The listing builds one solid part. Answer for the finished solid, in the listing's coordinates (mm). Face numbers are marked on the shaded views. A direction names the side the tool comes from. Round coordinates to 2 decimals unless told otherwise and drop trailing zeros. Loops run counter-clockwise (first coordinate to the right, second up) from the corner with the lowest first, then second, coordinate; pieces in that order, holes last. Notation, with made-up numbers: (12, 85.5) -> (20, 85.5) arc R29 ccw to (20, 113.5) -> close; hole circle Ø2 at (41, 45.25). An arc over 180 degrees is marked (long way). Answer in a Markdown table with one row per item. Add a question column.
```python
from build123d import *

# Parameters (mm, degrees)
BOSS_EXTRUDE1_DEPTH     = 22.4
FILLET1_R               = 2
FILLET2_R               = 5.5
BOSS_EXTRUDE2_DEPTH     = 2.73
CUT_EXTRUDE2_DEPTH      = 32.510198396
CUT_EXTRUDE2_DEPTH_BACK = 32.510198396
SKETCH3_R               = 0.95


with BuildPart() as part:
    # Sketch1 → Boss-Extrude1 (new body)
    with BuildSketch(Plane(origin=(0, 0, 0), x_dir=(1, 0, 0), z_dir=(0, 1, 0))):
        Polygon((-7.925386608, 7.925386608), (-15.2, -4.674613392), (-18.231088913, -2.924613392), (-9.94611255, 11.425386608), (9.94611255, 11.425386608), (18.231088913, -2.924613392), (15.2, -4.674613392), (7.925386608, 7.925386608), align=None)
    extrude(amount=BOSS_EXTRUDE1_DEPTH)

    # Fillet1
    fillet1_edges = [part.edges().sort_by_distance(p)[0] for p in [
        (7.925386608, 11.2, -7.925386608),
        (-7.925386608, 11.2, -7.925386608),
    ]]
    fillet(fillet1_edges, radius=FILLET1_R)

    # Fillet2
    fillet2_edges = [part.edges().sort_by_distance(p)[0] for p in [
        (-9.94611255, 11.2, -11.425386608),
        (9.94611255, 11.2, -11.425386608),
    ]]
    fillet(fillet2_edges, radius=FILLET2_R)

    # Sketch2 → Boss-Extrude2 (add)
    with BuildSketch(Plane.XY.offset(-7.925386608)):
        with BuildLine():
            Line((-0.32, 17.93), (0.32, 17.93))
            ThreePointArc((0.32, 17.93), (1.27, 16.98), (2.22, 17.93))
            Line((2.22, 17.93), (2.86, 17.93))
            ThreePointArc((2.86, 17.93), (3.138248558, 17.258248558), (3.81, 16.98))
            Line((3.81, 16.98), (3.81, 16.34))
            ThreePointArc((3.81, 16.34), (3.138248558, 16.061751442), (2.86, 15.39))
            Line((2.86, 15.39), (2.22, 15.39))
            ThreePointArc((2.22, 15.39), (1.27, 16.34), (0.32, 15.39))
            Line((0.32, 15.39), (-0.32, 15.39))
            ThreePointArc((-0.32, 15.39), (-1.27, 16.34), (-2.22, 15.39))
            Line((-2.22, 15.39), (-2.86, 15.39))
            ThreePointArc((-2.86, 15.39), (-3.138248558, 16.061751442), (-3.81, 16.34))
            Line((-3.81, 16.34), (-3.81, 16.98))
            ThreePointArc((-3.81, 16.98), (-3.138248558, 17.258248558), (-2.86, 17.93))
            Line((-2.86, 17.93), (-2.22, 17.93))
            ThreePointArc((-2.22, 17.93), (-1.27, 16.98), (-0.32, 17.93))
        make_face()
    extrude(amount=BOSS_EXTRUDE2_DEPTH)

    # Sketch3 → Cut-Extrude2 (cut, two sides: drawn at the far end of the back side and taken through both)
    with BuildSketch(Plane.XY.offset(-7.925386608).offset(-CUT_EXTRUDE2_DEPTH_BACK)):
        with Locations((-3.81, 17.93)):
            Circle(SKETCH3_R)
        with Locations((-1.27, 17.93)):
            Circle(SKETCH3_R)
        with Locations((1.27, 17.93)):
            Circle(SKETCH3_R)
        with Locations(Location((3.81, 17.93, 0), (0, 0, 180))):
            Circle(SKETCH3_R)
        with Locations(Location((3.81, 15.39, 0), (0, 0, 180))):
            Circle(SKETCH3_R)
        with Locations((1.27, 15.39)):
            Circle(SKETCH3_R)
        with Locations((-1.27, 15.39)):
            Circle(SKETCH3_R)
        with Locations((-3.81, 15.39)):
            Circle(SKETCH3_R)
    extrude(amount=CUT_EXTRUDE2_DEPTH + CUT_EXTRUDE2_DEPTH_BACK, mode=Mode.SUBTRACT)


solid = part.part
```
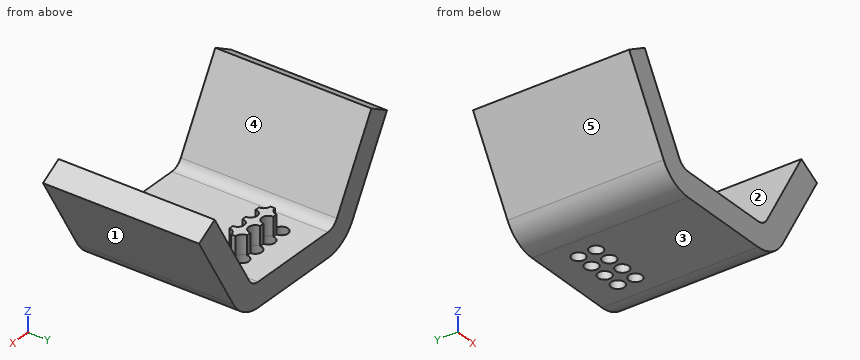
Item 1: Section C-C, the plane y = 1.5 is taken. Write down the section's boundary in (x, z).
Item 2: Consider L1, parallel to Y at x = -3.81, z = -9.35; L2, parallel to X at y = 15.39, z = -8.7; L3, parallel to X at y = 17.93, z = -9.15. Determine where each line is inside the solid, lowest interval first. Write a range as from..to.
Item 3: Section A-A, the plane x = 1.27 is taken. Write down the section's boundary in (y, z), and give its area (3 significant figures).
Item 4: The mould has two halves that part along X. Classify the marked faces 3, 4 and 5: +X half, -X half, draft (parallel to the pull), parting line (faces both ways), or undercut.
Item 5: Section B-B, the plane z = -1 is taken. Write down the section's boundary in (x, y).
Item 6: Flat-ended cylindrical pins translate along their axes: P1, Ø0.7, axis at x = -2.5, z = -7, coming from the +Y side; P2, Ø6, axis at x = -7.5, y = 9.5, coming from the +Z side; P3, Ø1, axis at x = -0.5, z = -5.5, coming from the -Y side; P4, Ø1.5, axis at x = 3.81, y = 17.93, coming from the +Z side. Find the tip coordinate at first contact, or state that the pin passes through.
Item 7: For the marked faces 1 and 2, determine the directions among +Z, -Z, +X, -X, +Y, -Y from which every point of the face is accessible in a straight line to the end or side of a thin tool.
Item 8: Section D-D, the plane y = 15 is taken. Write down the section's boundary in (x, z), and give its area (3 significant figures).
Here are the results:
| question | item | result |
|---|---|---|
| 1 | outline | (-18.23, 2.92) -> (-11.53, -8.68) arc R5.5 ccw to (-6.77, -11.43) -> (6.77, -11.43) arc R5.5 ccw to (11.53, -8.68) -> (18.23, 2.92) -> (15.2, 4.67) -> (8.5, -6.93) arc R2 cw to (6.77, -7.93) -> (-6.77, -7.93) arc R2 cw to (-8.5, -6.93) -> (-15.2, 4.67) -> close |
| 2 | L1 | y = 0..14.44, 16.34..16.98, 18.88..22.4 |
| 2 | L2 | x = -11.52..-4.76, -2.86..-2.22, -0.32..0.32, 2.22..2.86, 4.76..11.52 |
| 2 | L3 | x = -11.23..-4.76, -2.86..-2.22, -0.32..0.32, 2.22..2.86, 4.76..11.23 |
| 3 | outline | (0, -11.43) -> (14.44, -11.43) -> (14.44, -7.93) -> (0, -7.93) -> close; (16.34, -11.43) -> (16.98, -11.43) -> (16.98, -5.2) -> (16.34, -5.2) -> close; (18.88, -11.43) -> (22.4, -11.43) -> (22.4, -7.93) -> (18.88, -7.93) -> close |
| 3 | area | 66.8 mm² |
| 4 | face 3 | draft |
| 4 | face 4 | undercut |
| 4 | face 5 | -X half |
| 5 | outline | (-15.97, 0) -> (-11.92, 0) -> (-11.92, 22.4) -> (-15.97, 22.4) -> close; (11.92, 0) -> (15.97, 0) -> (15.97, 22.4) -> (11.92, 22.4) -> close |
| 6 | P1 | stops at y = 17.93 |
| 6 | P2 | stops at z = -3.47 |
| 6 | P3 | stops at y = 15.39 |
| 6 | P4 | passes through |
| 7 | face 1 | -Z, +X, +Y, -Y |
| 7 | face 2 | +Z, +Y, -Y |
| 8 | outline | (-18.23, 2.92) -> (-11.53, -8.68) arc R5.5 ccw to (-6.77, -11.43) -> (-4.68, -11.43) -> (-4.68, -7.93) -> (-6.77, -7.93) arc R2 cw to (-8.5, -6.93) -> (-15.2, 4.67) -> close; (-2.94, -11.43) -> (-2.14, -11.43) -> (-2.14, -7.93) -> (-2.94, -7.93) -> close; (-0.4, -11.43) -> (0.4, -11.43) -> (0.4, -7.93) -> (-0.4, -7.93) -> close; (2.14, -11.43) -> (2.94, -11.43) -> (2.94, -7.93) -> (2.14, -7.93) -> close; (4.68, -11.43) -> (6.77, -11.43) arc R5.5 ccw to (11.53, -8.68) -> (18.23, 2.92) -> (15.2, 4.67) -> (8.5, -6.93) arc R2 cw to (6.77, -7.93) -> (4.68, -7.93) -> close |
| 8 | area | 144 mm² |
